from build123d import *

# Parameters (mm, degrees)
RESSALTO_EXTRUS_O1_DEPTH      = 12
RESSALTO_EXTRUS_O1_DEPTH_BACK = 12
ESBO_O1_W                     = 175
ESBO_O1_H                     = 90
CORTE_EXTRUS_O1_DEPTH         = 198.15222545
CORTE_EXTRUS_O1_DEPTH_BACK    = 198.15222545
ESBO_O3_W                     = 150
ESBO_O3_H                     = 15
CORTE_EXTRUS_O2_DEPTH         = 198.15222545
CORTE_EXTRUS_O2_DEPTH_BACK    = 198.15222545
ESBO_O4_R                     = 7.5
FILETE1_R                     = 3.5
FILETE2_R                     = 3.5
FILETE3_R                     = 3.5


with BuildPart() as part:
    # Esboço1 → Ressalto-extrusão1 (new, two sides: drawn at the far end of the back side and taken through both)
    with BuildSketch(Plane.XY.offset(-RESSALTO_EXTRUS_O1_DEPTH_BACK)):
        with Locations((87.5, 45)):
            Rectangle(ESBO_O1_W, ESBO_O1_H)
    extrude(amount=RESSALTO_EXTRUS_O1_DEPTH + RESSALTO_EXTRUS_O1_DEPTH_BACK)

    # Esboço3 → Corte-extrusão1 (cut, two sides: drawn at the far end of the back side and taken through both)
    with BuildSketch(Plane(origin=(0, 0, 0), x_dir=(1, 0, 0), z_dir=(0, 1, 0)).offset(-CORTE_EXTRUS_O1_DEPTH_BACK)):
        with Locations((100, 4.5)):
            Rectangle(ESBO_O3_W, ESBO_O3_H)
    extrude(amount=CORTE_EXTRUS_O1_DEPTH + CORTE_EXTRUS_O1_DEPTH_BACK, mode=Mode.SUBTRACT)

    # Esboço4 → Corte-extrusão2 (cut, two sides: drawn at the far end of the back side and taken through both)
    with BuildSketch(Plane(origin=(0, 90, 0), x_dir=(1, 0, 0), z_dir=(0, 1, 0)).offset(-CORTE_EXTRUS_O2_DEPTH_BACK)):
        with Locations(Location((12.5, 0, 0), (0, 0, 270))):
            Circle(ESBO_O4_R)
    extrude(amount=CORTE_EXTRUS_O2_DEPTH + CORTE_EXTRUS_O2_DEPTH_BACK, mode=Mode.SUBTRACT)

    # Filete1
    filete1_edges = [part.edges().sort_by_distance(p)[0] for p in [
        (25, 45, -12),
        (25, 45, 3),
        (0, 45, -12),
    ]]
    fillet(filete1_edges, radius=FILETE1_R)

    # Filete2
    filete2_edges = [part.edges().sort_by_distance(p)[0] for p in [
        (175, 45, 12),
        (87.5, 90, 12),
        (175, 45, 3),
    ]]
    fillet(filete2_edges, radius=FILETE2_R)

    # Filete3
    # the kernel refuses this fillet: 3.5 mm, written as the material it takes off along each edge
    with BuildSketch(Plane(origin=(171.5, 86.5, 8.5), x_dir=(0, 1, 0), z_dir=(1, 0, 0))) as filete3_piece_1_section:
        Polygon((0, 0), (FILETE3_R, 0), (FILETE3_R, FILETE3_R), (0, FILETE3_R), align=None)
    filete3_piece_1 = extrude(amount=FILETE3_R, mode=Mode.PRIVATE)
    filete3_piece_1 = filete3_piece_1 - Plane(origin=(171.5, 86.5, 8.5), x_dir=(0, -0.7071067811865475, -0.7071067811865475), z_dir=(1, 0, 0)) * Sphere(FILETE3_R, mode=Mode.PRIVATE)
    add(filete3_piece_1, mode=Mode.SUBTRACT)
    with BuildSketch(Plane(origin=(3.5, 3.5, 8.5), x_dir=(0, 0, 1), z_dir=(0, -1, 0))) as filete3_piece_2_section:
        Polygon((0, 0), (FILETE3_R, 0), (FILETE3_R, FILETE3_R), (0, FILETE3_R), align=None)
    filete3_piece_2 = extrude(amount=FILETE3_R, mode=Mode.PRIVATE)
    filete3_piece_2 = filete3_piece_2 - Plane(origin=(3.5, 3.5, 8.5), x_dir=(0.7071067811865475, 0, -0.7071067811865475), z_dir=(0, -1, 0)) * Sphere(FILETE3_R, mode=Mode.PRIVATE)
    add(filete3_piece_2, mode=Mode.SUBTRACT)
    with BuildSketch(Plane(origin=(3.5, 0, 12), x_dir=(0, 0, -1), z_dir=(1, 0, 0))) as filete3_piece_3:
        with BuildLine():
            CenterArc((FILETE3_R, FILETE3_R), FILETE3_R, 180, 90)
            Line((0, FILETE3_R), (0, 0))
            Line((0, 0), (FILETE3_R, 0))
        make_face()
    extrude(amount=168, mode=Mode.SUBTRACT)
    with BuildSketch(Plane(origin=(0, 0, 8.5), x_dir=(1, 0, 0), z_dir=(0, 0, -1)), Plane(origin=(0, 90, 8.5), x_dir=(0, -1, 0), z_dir=(0, 0, -1))) as filete3_piece_4:
        with BuildLine():
            CenterArc((FILETE3_R, -FILETE3_R), FILETE3_R, 90, 90)
            Line((0, -FILETE3_R), (0, 0))
            Line((0, 0), (FILETE3_R, 0))
        make_face()
    extrude(amount=17, mode=Mode.SUBTRACT)
    with BuildSketch(Plane(origin=(25, 0, -8.5), x_dir=(-1, 0, 0), z_dir=(0, 0, 1))) as filete3_piece_5:
        with BuildLine():
            CenterArc((FILETE3_R, -FILETE3_R), FILETE3_R, 90, 90)
            Line((0, -FILETE3_R), (0, 0))
            Line((0, 0), (FILETE3_R, 0))
        make_face()
    extrude(amount=8, mode=Mode.SUBTRACT)
    with BuildSketch(Plane(origin=(3.5, 0, -12), x_dir=(0, 0, 1), z_dir=(1, 0, 0))) as filete3_piece_6:
        with BuildLine():
            CenterArc((FILETE3_R, -FILETE3_R), FILETE3_R, 90, 90)
            Line((0, -FILETE3_R), (0, 0))
            Line((0, 0), (FILETE3_R, 0))
        make_face()
    extrude(amount=18, mode=Mode.SUBTRACT)
    with BuildSketch(Plane(origin=(21.5, 0, -8.5), x_dir=(0, 0, -1), z_dir=(-1, 0, 0))) as filete3_piece_7:
        with BuildLine():
            CenterArc((3.5 - FILETE3_R, -FILETE3_R), FILETE3_R, 0, 90)
            Line((3.5, -FILETE3_R), (3.5, 0))
            Line((3.5, 0), (3.5 - FILETE3_R, 0))
        make_face()
    revolve(axis=Axis((21.5, 0, -8.5), (0, -1, 0)), revolution_arc=90, mode=Mode.SUBTRACT)
    with BuildSketch(Plane(origin=(3.5, 0, -8.5), x_dir=(-1, 0, 0), z_dir=(0, 0, 1))) as filete3_piece_8:
        with BuildLine():
            CenterArc((3.5 - FILETE3_R, -FILETE3_R), FILETE3_R, 0, 90)
            Line((3.5, -FILETE3_R), (3.5, 0))
            Line((3.5, 0), (3.5 - FILETE3_R, 0))
        make_face()
    revolve(axis=Axis((3.5, 0, -8.5), (0, -1, 0)), revolution_arc=90, mode=Mode.SUBTRACT)
    with BuildSketch(Plane(origin=(21.5, 90, -12), x_dir=(0, -1, 0), z_dir=(-1, 0, 0))) as filete3_piece_9:
        with BuildLine():
            CenterArc((FILETE3_R, FILETE3_R), FILETE3_R, 180, 90)
            Line((0, FILETE3_R), (0, 0))
            Line((0, 0), (FILETE3_R, 0))
        make_face()
    extrude(amount=18, mode=Mode.SUBTRACT)
    with BuildSketch(Plane(origin=(25, 90, -0.5), x_dir=(0, -1, 0), z_dir=(0, 0, -1))) as filete3_piece_10:
        with BuildLine():
            CenterArc((FILETE3_R, FILETE3_R), FILETE3_R, 180, 90)
            Line((0, FILETE3_R), (0, 0))
            Line((0, 0), (FILETE3_R, 0))
        make_face()
    extrude(amount=8, mode=Mode.SUBTRACT)
    with BuildSketch(Plane(origin=(171.5, 90, 3), x_dir=(0, -1, 0), z_dir=(-1, 0, 0))) as filete3_piece_11:
        with BuildLine():
            CenterArc((FILETE3_R, FILETE3_R), FILETE3_R, 180, 90)
            Line((0, FILETE3_R), (0, 0))
            Line((0, 0), (FILETE3_R, 0))
        make_face()
    extrude(amount=143, mode=Mode.SUBTRACT)
    with BuildSketch(Plane(origin=(21.5, 90, -8.5), x_dir=(0, 0, -1), z_dir=(-1, 0, 0))) as filete3_piece_12:
        with BuildLine():
            CenterArc((3.5 - FILETE3_R, FILETE3_R), FILETE3_R, 270, 90)
            Line((3.5 - FILETE3_R, 0), (3.5, 0))
            Line((3.5, 0), (3.5, FILETE3_R))
        make_face()
    revolve(axis=Axis((21.5, 90, -8.5), (0, -1, 0)), revolution_arc=90, mode=Mode.SUBTRACT)
    with BuildSketch(Plane(origin=(3.5, 90, -8.5), x_dir=(-1, 0, 0), z_dir=(0, 0, 1))) as filete3_piece_13:
        with BuildLine():
            CenterArc((3.5 - FILETE3_R, FILETE3_R), FILETE3_R, 270, 90)
            Line((3.5 - FILETE3_R, 0), (3.5, 0))
            Line((3.5, 0), (3.5, FILETE3_R))
        make_face()
    revolve(axis=Axis((3.5, 90, -8.5), (0, -1, 0)), revolution_arc=90, mode=Mode.SUBTRACT)
    with BuildSketch(Plane(origin=(28.5, 90, -0.5), x_dir=(-1, 0, 0), z_dir=(0, 0, -1))) as filete3_piece_14:
        with BuildLine():
            CenterArc((3.5 + FILETE3_R, -FILETE3_R), FILETE3_R, 90, 90)
            Line((3.5 + FILETE3_R, 0), (3.5, 0))
            Line((3.5, 0), (3.5, -FILETE3_R))
        make_face()
    revolve(axis=Axis((28.5, 90, -0.5), (0, 1, 0)), revolution_arc=90, mode=Mode.SUBTRACT)
    with BuildSketch(Plane(origin=(28.5, 0, -0.5), x_dir=(-1, 0, 0), z_dir=(0, 0, -1))) as filete3_piece_15:
        with BuildLine():
            CenterArc((3.5 + FILETE3_R, FILETE3_R), FILETE3_R, 180, 90)
            Line((3.5, FILETE3_R), (3.5, 0))
            Line((3.5, 0), (3.5 + FILETE3_R, 0))
        make_face()
    revolve(axis=Axis((28.5, 0, -0.5), (0, 1, 0)), revolution_arc=90, mode=Mode.SUBTRACT)
    with BuildSketch(Plane(origin=(0, 86.5, 12), x_dir=(1, 0, 0), z_dir=(0, -1, 0))) as filete3_piece_16:
        with BuildLine():
            CenterArc((FILETE3_R, -FILETE3_R), FILETE3_R, 90, 90)
            Line((0, -FILETE3_R), (0, 0))
            Line((0, 0), (FILETE3_R, 0))
        make_face()
    extrude(amount=83, mode=Mode.SUBTRACT)
    with BuildSketch(Plane(origin=(0, 86.5, 8.5), x_dir=(0, 0, 1), z_dir=(0, -1, 0))) as filete3_piece_17:
        with BuildLine():
            CenterArc((3.5 - FILETE3_R, -FILETE3_R), FILETE3_R, 0, 90)
            Line((3.5, -FILETE3_R), (3.5, 0))
            Line((3.5, 0), (3.5 - FILETE3_R, 0))
        make_face()
    revolve(axis=Axis((0, 86.5, 8.5), (-1, 0, 0)), revolution_arc=90, mode=Mode.SUBTRACT)
    with BuildSketch(Plane(origin=(175, 90, 6.5), x_dir=(0, -1, 0), z_dir=(0, 0, 1)), Plane(origin=(175, 0, 6.5), x_dir=(-1, 0, 0), z_dir=(0, 0, 1))) as filete3_piece_18:
        with BuildLine():
            CenterArc((FILETE3_R, -FILETE3_R), FILETE3_R, 90, 90)
            Line((0, -FILETE3_R), (0, 0))
            Line((0, 0), (FILETE3_R, 0))
        make_face()
    extrude(amount=2, mode=Mode.SUBTRACT)
    with BuildSketch(Plane(origin=(171.5, 90, 6.5), x_dir=(1, 0, 0), z_dir=(0, 0, 1))) as filete3_piece_19:
        with BuildLine():
            CenterArc((3.5 - FILETE3_R, -FILETE3_R), FILETE3_R, 0, 90)
            Line((3.5 - FILETE3_R, 0), (3.5, 0))
            Line((3.5, 0), (3.5, -FILETE3_R))
        make_face()
    revolve(axis=Axis((171.5, 90, 6.5), (0, 1, 0)), revolution_arc=90, mode=Mode.SUBTRACT)
    with BuildSketch(Plane(origin=(28.5, 0, 3), x_dir=(0, 0, 1), z_dir=(1, 0, 0))) as filete3_piece_20:
        with BuildLine():
            CenterArc((FILETE3_R, -FILETE3_R), FILETE3_R, 90, 90)
            Line((0, -FILETE3_R), (0, 0))
            Line((0, 0), (FILETE3_R, 0))
        make_face()
    extrude(amount=143, mode=Mode.SUBTRACT)
    with BuildSketch(Plane(origin=(171.5, 0, 6.5), x_dir=(1, 0, 0), z_dir=(0, 0, 1))) as filete3_piece_21:
        with BuildLine():
            CenterArc((3.5 - FILETE3_R, FILETE3_R), FILETE3_R, 270, 90)
            Line((3.5, FILETE3_R), (3.5, 0))
            Line((3.5, 0), (3.5 - FILETE3_R, 0))
        make_face()
    revolve(axis=Axis((171.5, 0, 6.5), (0, 1, 0)), revolution_arc=90, mode=Mode.SUBTRACT)
    with BuildSketch(Plane(origin=(171.5, 0, 8.5), x_dir=(0, 0, 1), z_dir=(-1, 0, 0))) as filete3_piece_22:
        with BuildLine():
            CenterArc((3.5 - FILETE3_R, FILETE3_R), FILETE3_R, 270, 90)
            Line((3.5, FILETE3_R), (3.5, 0))
            Line((3.5, 0), (3.5 - FILETE3_R, 0))
        make_face()
    revolve(axis=Axis((171.5, 0, 8.5), (0, 1, 0)), revolution_arc=90, mode=Mode.SUBTRACT)


solid = part.part
The listing builds one solid part. Answer for the finished solid, in the listing's coordinates (mm). A direction names the side the tool comes from. Give positions to 0.01 mm unless a question says otherwise; leave off trailing zeros. Write each loop counter-clockwise with the first axis right and the second up, starting at its lowest first coordinate (ties: lowest second). Pieces come first, ordered by that corner, then holes. Notation, with made-up numbers: (15, 58.25) - (29, 58.25) arc R15 cw to (29, 69.25) - close; hole circle Ø1 at (81.5, -35). An arc over 180 degrees is marked (long way). One line per question, with ' | ' between items. Start each with the question number.
1. Section A-A, the plane x = 12.5 is taken. Determine the outline of the cut face in (y, z), then the cut area to 3 significant figures.
2. For faces 4 (the face through (25, 44, -4)), 5 (the face through (23.95, 89, -4.44)), 6 (the face through (23.95, 1, -4.56)), determine the directions among +Z, -Z, +X, -X, +Y, -Y from which every point of the face is accessible in a straight line to the end or side of a thin tool.
3. Determine the mould class of faces 1 (the face through (101, 89, 4.05)), 2 (the face through (1.05, 45.58, 11)), 3 (the face through (174, 45.58, 4.05)) for opening direction X: +X half, -X half, draft (parallel to the pull), parting line (faces both ways), or undercut.
4. Given P1, Ø10, axis at x = 57, z = 7.5, coming from the -Y side; P2, Ø2, axis at y = 11.5, z = -2.5, coming from the +X side, each flat-ended and moving along its own axis, determine where each tip first touches the part or whether it passes through.
5. Section C-C, the plane z = -5.25 is taken. Determine the outline of the cut face in (x, y).
6. Section D-D, the plane x = 142 is taken. Determine the outline of the cut face in (y, z).
7. Straight lines are drawn through the part: line 1 (Z direction, x = 12.5, y = 45); line 2 (X direction, y = 38, z = 0); line 3 (Z direction, x = 116, y = 50). For each, find the intervals that lie inside material, in ascending order.
8. Section B-B, the plane y = 66.5 is taken. Determine the outline of the cut face in (x, z), then the cut area to 3 significant figures.
Result:
1) outline: (0, -8.5) arc R3.5 ccw to (3.5, -12) - (86.5, -12) arc R3.5 ccw to (90, -8.5) - (90, -7.5) - (0, -7.5) - close; (0, 7.5) - (90, 7.5) - (90, 8.5) arc R3.5 ccw to (86.5, 12) - (3.5, 12) arc R3.5 ccw to (0, 8.5) - close | area: 799 mm2
2) face 4: -Z, +X, +Y, -Y | face 5: -Z, +X, +Y | face 6: -Z, +X, -Y
3) face 1: draft | face 2: -X half | face 3: +X half
4) P1: stops at y = 0 | P2: stops at x = 25
5) outline: (0, 3.5) arc R3.5 ccw to (3.5, 0) - (7.14, 0) - (7.14, 90) - (3.5, 90) arc R3.5 ccw to (0, 86.5) - close; (17.86, 0) - (21.5, 0) arc R3.5 ccw to (25, 3.5) - (25, 86.5) arc R3.5 ccw to (21.5, 90) - (17.86, 90) - close
6) outline: (0, 6.5) arc R3.5 ccw to (3.5, 3) - (86.5, 3) arc R3.5 ccw to (90, 6.5) - (90, 8.5) arc R3.5 ccw to (86.5, 12) - (3.5, 12) arc R3.5 ccw to (0, 8.5) - close
7) line 1: z = -12 to -7.5, 7.5 to 12 | line 2: x = 0 to 5, 20 to 25.04 | line 3: z = 3 to 12
8) outline: (0, -8.5) arc R3.5 ccw to (3.5, -12) - (21.5, -12) arc R3.5 ccw to (25, -8.5) - (25, -0.5) arc R3.5 cw to (28.5, 3) - (171.5, 3) arc R3.5 ccw to (175, 6.5) - (175, 8.5) arc R3.5 ccw to (171.5, 12) - (3.5, 12) arc R3.5 ccw to (0, 8.5) - close; hole circle Ø15 at (12.5, 0) | area: 1,760 mm2
